Autodesk Inventor part; units mm, degrees
ref_plane "YZ Plane" through (0, 0, 0) normal (1, 0, 0) x (0, 1, 0)
ref_plane "XZ Plane" through (0, 0, 0) normal (0, 1, 0) x (-1, 0, 0)
ref_plane "XY Plane" through (0, 0, 0) normal (0, 0, 1) x (1, 0, 0)
sketch "Sketch1" plane through (0, 0, 0) normal (0, 0, 1) x (1, 0, 0)
  line L0 (-10, -30) -> (10, -30)
  line L1 (10, -30) -> (10, 30)
  line L2 (10, 30) -> (-10, 30)
  line L3 (-10, 30) -> (-10, -30)
  line L4 (-10, -30) -> (10, 30) construction
  line L5 (10, -30) -> (-10, 30) construction
  circle A0 centre (1.5, 20) radius 2.75
  circle A1 centre (1.5, -20) radius 2.75
  point P0 (0, 0)
  dimension "d0" = 20
  dimension "d1" = 60
  dimension "d20" = 5.5
  dimension "d21" = 5.5
  dimension "d22" = 10
  dimension "d23" = 8.5
  dimension "d24" = 8.5
  dimension "d25" = 10
extrude "Extrusion1" add sketch "Sketch1" along normal blind 3
sketch "Sketch2" plane through (0, 0, 3) normal (0, 0, 1) x (1, 0, 0)
  line L0 (10, 30) -> (-10, 30)
  line L1 (-10, 30) -> (-7, 30)
  line L2 (-7, 30) -> (-7, -30)
  line L3 (-7, -30) -> (-10, -30)
  line L4 (-10, -30) -> (-10, 30)
  point P0 (0, 0)
  dimension "d4" = 3
  dimension "d5" = 60
extrude "Extrusion2" add sketch "Sketch2" along normal blind 17
sketch "Sketch3" plane through (-10, 30, 0) normal (0, 1, 0) x (1, 0, 0)
  line L0 (0, 0) -> (20, 0)
  line L1 (20, 0) -> (20, -20)
  line L2 (20, -20) -> (0, -20)
  line L3 (0, -20) -> (0, 0)
  point P0 (10, 0)
  dimension "d8" = 20
  dimension "d9" = 20
extrude "Extrusion3" add sketch "Sketch3" against normal blind 3
sketch "Sketch4" plane through (-10, -30, 0) normal (0, -1, 0) x (1, 0, 0)
  line L0 (0, 0) -> (20, 0)
  line L1 (20, 0) -> (20, 20)
  line L2 (20, 20) -> (0, 20)
  line L3 (0, 20) -> (0, 0)
  point P0 (10, 0)
  dimension "d12" = 20
  dimension "d13" = 20
extrude "Extrusion4" add sketch "Sketch4" against normal blind 3
chamfer "Chamfer1" distance 17 angle 45 2 edges at (10, -28.5, 20) (10, 28.5, 20)
fillet "Fillet1" radius 2 2 edges at (1.5, 27, 3) (1.5, -27, 3)
sketch "Sketch5" plane through (-7, -27, 20) normal (1, 0, 0) x (0, 0, -1)
  circle A0 centre (8.5, 7) radius 2.75
  circle A1 centre (8.5, 47) radius 2.75
  line L0 (17, 57) -> (0, 57)
  line L1 (0, 0) -> (0, 54)
  line L2 (0, -3) -> (17, -3)
  point P0 (20, 27)
  dimension "d26" = 5.5
  dimension "d27" = 5.5
  dimension "d28" = 10
  dimension "d29" = 8.5
  dimension "d30" = 8.5
  dimension "d31" = 10
extrude "Extrusion5" cut sketch "Sketch5" against normal blind 3
properties part number "2060 Custom Bracing" material "Aluminum 6061"
Input: part model. Units: mm. Frame: model coordinates. A direction names the side the tool comes from. Coordinates: 2 decimals unless noted, no trailing zeros. Loops run counter-clockwise (first coordinate to the right, second up) from the corner with the lowest first, then second, coordinate; pieces in that order, holes last. Notation, with made-up numbers: (76, 75) -> (106, 75) arc R21 cw to (106, 91) -> close; hole circle Ø2 at (6, 12). An arc over 180 degrees is marked (long way). Write each question's results on one line, items separated by ' | '. Start each with the question number.
Q1. Section D-D, the plane z = 15.25. Return the cut outline in (x, y).
Q2. Ray query, line 1 (Y direction, x = -8, z = 11.5); line 2 (Y direction, x = -6.5, z = 19.25); line 3 (Z direction, x = -4.25, y = 2). Return the intervals inside material, ascending. Write a range as from..to.
Q3. Section C-C, the plane x = 1.5. Return the cut outline in (y, z).
Q4. Section B-B, the plane y = 20. Return the cut outline in (x, z).
Q5. Pull-direction query (Z, two-part tool) for faces 3 (the cylindrical face through (-8.479, -17.273, 11.858)), 4 (the flat face through (2, -29, 11)), 5 (the flat face through (-3, -27, 9)), 6 (the flat face through (0, 0, 0)); classes: released by +Z, released by -Z, zero draft, split by the parting line, or undercut.
Q6. Section A-A, the plane z = 11.5. Return the cut outline in (x, y), plus the area to 3 significant figures.
Q7. Pin query (flat end, axial travel): pin 1 (5 mm diameter, centred on x = -2.5, y = -13.5, fed in from +Z); pin 2 (8.5 mm diameter, centred on y = 8, z = 7.5, fed in from +X); pin 3 (12 mm diameter, centred on y = -22, z = 12.5, fed in from -X). Return the tip coordinate at first contact, or that it passes through.
Q8. Reachability of faces 1 (the cylindrical face through (1.62, -26.43, 3.6)), 2 (the flat face through (2, 29, 11)) from +Z, -Z, +X, -X, +Y, -Y: full face, straight path, thin tool, end or side. Return the list, or none.
Found:
1) outline: (-10, -30) -> (-2.25, -30) -> (-2.25, -27) -> (-7, -27) -> (-7, 27) -> (-2.25, 27) -> (-2.25, 30) -> (-10, 30) -> close
2) line 1: -30..-22.75, -17.25..17.25, 22.75..30 | line 2: -30..-27, 27..30 | line 3: 0..3
3) outline: (-30, 0) -> (-22.75, 0) -> (-22.75, 3) -> (-25, 3) arc R2 cw to (-27, 5) -> (-27, 11.5) -> (-30, 11.5) -> close; (-17.25, 0) -> (17.25, 0) -> (17.25, 3) -> (-17.25, 3) -> close; (22.75, 0) -> (30, 0) -> (30, 11.5) -> (27, 11.5) -> (27, 5) arc R2 cw to (25, 3) -> (22.75, 3) -> close
4) outline: (-10, 0) -> (-1.25, 0) -> (-1.25, 3) -> (-7, 3) -> (-7, 8.75) -> (-10, 8.75) -> close; (-10, 14.25) -> (-7, 14.25) -> (-7, 20) -> (-10, 20) -> close; (4.25, 0) -> (10, 0) -> (10, 3) -> (4.25, 3) -> close
5) face 3: undercut | face 4: released by +Z | face 5: zero draft | face 6: released by -Z
6) outline: (-10, -30) -> (1.5, -30) -> (1.5, -27) -> (-7, -27) -> (-7, -22.75) -> (-10, -22.75) -> close; (-10, -17.25) -> (-7, -17.25) -> (-7, 17.25) -> (-10, 17.25) -> close; (-10, 22.75) -> (-7, 22.75) -> (-7, 27) -> (1.5, 27) -> (1.5, 30) -> (-10, 30) -> close | area: 198 mm2
7) pin 1: z = 3 | pin 2: x = -7 | pin 3: x = -10
8) face 1: +Z, +X | face 2: +Z, +X, +Y, -Y
